Read the model definition and answer for the solid it produces. Units are mm, in the model's axes. Face numbers are marked on the shaded views. A direction names the side the tool comes from. Coordinates: 2 decimals unless noted, no trailing zeros. Write each loop counter-clockwise with the first axis right and the second up, starting at its lowest first coordinate (ties: lowest second). Pieces come first, ordered by that corner, then holes.
(1) The part is cut by section B-B, the plane x = 22. Determine the outline of the cut face in (y, z), and give its area (3 significant figures).
(2) The part is cut by section C-C, the plane z = 33.5. Determine the outline of the cut face in (x, y), and give its area (3 significant figures).
(3) The part is cut by section A-A, the plane y = 0. Determine the outline of the cut face in (x, z).
(4) Which of the six approach directions +Z, -Z, +X, -X, +Y, -Y give full straight-line access (tool end or side, diameter ignored) to the marked faces 1 and 2?
(5) Determine the mould class of the marked faces 3, 4, 5 and 6 for opening direction Y: pulls with the +Y half, pulls with the -Y half, needs draft (parallel to the pull), parting line crosses it, or undercut.
(6) Straight lines are drawn through the part: line 1 along Y through (x, z) = (0, 3.5); line 2 along Z through (x, y) = (43.5, -10); line 3 along X through (y, z) = (-19.5, 15). For each, find the intervals that lie inside material, in ascending order.
(7) Given pin 1 (5 mm diameter, centred on y = 8.5, z = 33.5, fed in from -X); pin 2 (17.5 mm diameter, centred on x = 6.5, y = 8.5, fed in from +Z); pin 3 (22.5 mm diameter, centred on x = 2.5, y = 2.5, fed in from +Z), each flat-ended and moving along its own axis, determine where each tip first touches the part or whether it passes through.
Autodesk Inventor part; units mm, degrees
ref_plane "YZ Plane" through (0, 0, 0) normal (1, 0, 0) x (0, 1, 0)
ref_plane "XZ Plane" through (0, 0, 0) normal (0, 1, 0) x (-1, 0, 0)
ref_plane "XY Plane" through (0, 0, 0) normal (0, 0, 1) x (1, 0, 0)
sketch "Schizzo1" plane through (0, 0, 0) normal (0, 0, 1) x (1, 0, 0)
  arc A0 (0, 22.5) -> (0, -22.5) centre (0, 0) ccw
  line L0 (0, 22.5) -> (45, 22.5)
  line L1 (45, 22.5) -> (45, -22.5)
  line L2 (45, -22.5) -> (0, -22.5)
  dimension "d1" = 45
  dimension "d2" = 45
extrude "Estrusione1" add sketch "Schizzo1" along normal blind 12
sketch "Schizzo2" plane through (0, 0, 12) normal (0, 0, 1) x (1, 0, 0)
  circle A0 centre (0, 0) radius 17.5
  dimension "d5" = 35
extrude "Estrusione2" cut sketch "Schizzo2" against normal blind 11
sketch "Schizzo3" plane through (0, 0, 1) normal (0, 0, 1) x (1, 0, 0)
  circle A0 centre (0, 0) radius 15.5
  dimension "d8" = 31
extrude "Estrusione3" cut sketch "Schizzo3" against normal up to next
chamfer "Smusso1" distance 0.5 angle 45 1 edges at (-17.5, 0, 12)
sketch "Schizzo4" plane through (45, -22.5, 0) normal (1, 0, 0) x (0, 0, -1)
  line L0 (0, 45) -> (0, 0)
  line L1 (0, 45) -> (-50, 45)
  line L2 (-50, 45) -> (-50, 0)
  line L3 (-50, 0) -> (0, 0)
  line L4 (0, 0) -> (0, 45)
  point P0 (0, 22.5)
  dimension "d15" = 50
  dimension "d16" = 45
extrude "Estrusione4" add sketch "Schizzo4" along normal blind 8
fillet "Raccordo2" radius 2 2 edges at (49, 22.5, 50) (49, -22.5, 50)
properties part number "Porta cuscinetto perno telaietto"
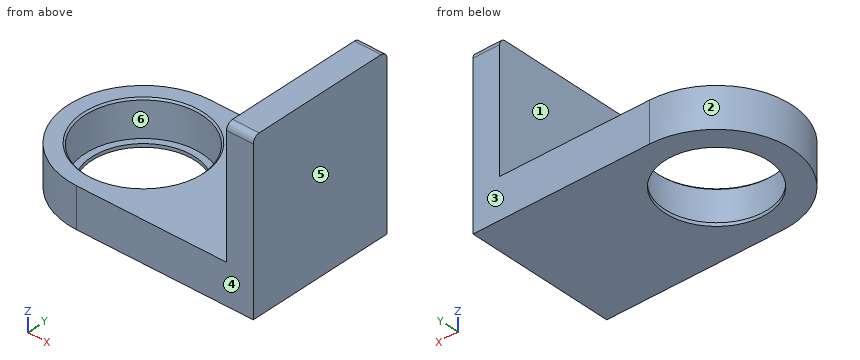
Computed:
1. outline: (-22.5, 0) - (22.5, 0) - (22.5, 12) - (-22.5, 12) - close
1. area: 540 mm2
2. outline: (45, -22.5) - (53, -22.5) - (53, 22.5) - (45, 22.5) - close
2. area: 360 mm2
3. outline: (-22.5, 0) - (-15.5, 0) - (-15.5, 1) - (-17.5, 1) - (-17.5, 11.5) - (-18, 12) - (-22.5, 12) - close; (15.5, 0) - (53, 0) - (53, 50) - (45, 50) - (45, 12) - (18, 12) - (17.5, 11.5) - (17.5, 1) - (15.5, 1) - close
4. face 1: +Z, -X, +Y, -Y
4. face 2: +Z, -Z, -X
5. face 3: pulls with the +Y half
5. face 4: pulls with the -Y half
5. face 5: needs draft
5. face 6: undercut
6. line 1: y = -22.5 to -17.5, 17.5 to 22.5
6. line 2: z = 0 to 12
6. line 3: x = 45 to 53
7. pin 1: stops at x = 45
7. pin 2: stops at z = 12
7. pin 3: passes through
